Geometry check sheet. Reference: the model listing, model coordinates, mm. Face numbers are marked on the shaded views. Give positions to 0.01 mm unless a question says otherwise; leave off trailing zeros. Write each loop counter-clockwise with the first axis right and the second up, starting at its lowest first coordinate (ties: lowest second). Pieces come first, ordered by that corner, then holes. Notation, with made-up numbers: (23.25, -24.75) - (80.25, -24.75) arc R29 ccw to (80.25, 6.25) - close; hole circle Ø11 at (82.5, -18). An arc over 180 degrees is marked (long way). Use a Markdown table: item, result.
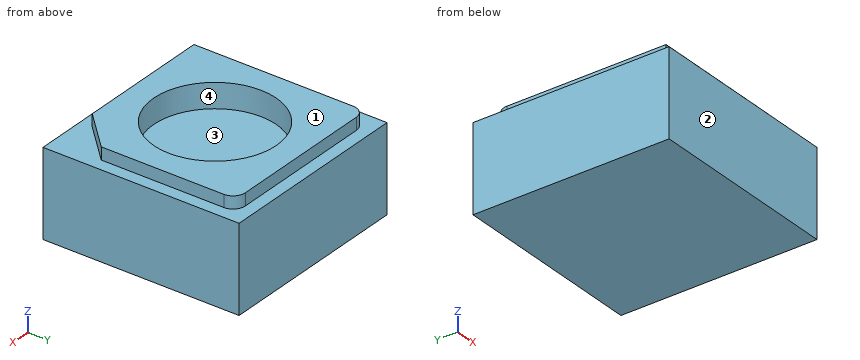
```python
from build123d import *

# Parameters (mm, degrees)
SKETCH1_W           = 80
SKETCH1_H           = 80
BOSS_EXTRUDE1_DEPTH = 35
BOSS_EXTRUDE2_START = 35
BOSS_EXTRUDE2_DEPTH = 5
CUT_EXTRUDE1_START  = 40
SKETCH3_R           = 25
CUT_EXTRUDE1_DEPTH  = 10


with BuildPart() as part:
    # Sketch1 → Boss-Extrude1 (new body)
    with BuildSketch(Plane.XY):
        with Locations((40, 40)):
            Rectangle(SKETCH1_W, SKETCH1_H)
    extrude(amount=BOSS_EXTRUDE1_DEPTH)

    # Sketch2 → Boss-Extrude2 (add)
    with BuildSketch(Plane.XY.offset(BOSS_EXTRUDE2_START)):
        with BuildLine():
            Line((60, 5), (75, 20))
            Line((75, 20), (75, 70))
            ThreePointArc((75, 70), (73.535533906, 73.535533906), (70, 75))
            Line((70, 75), (10, 75))
            ThreePointArc((10, 75), (6.464466094, 73.535533906), (5, 70))
            Line((5, 70), (5, 5))
            Line((5, 5), (60, 5))
        make_face()
    extrude(amount=BOSS_EXTRUDE2_DEPTH)

    # Sketch3 → Cut-Extrude1 (cut)
    with BuildSketch(Plane.XY.offset(CUT_EXTRUDE1_START)):
        with Locations((40, 40)):
            Circle(SKETCH3_R)
    extrude(amount=-CUT_EXTRUDE1_DEPTH, mode=Mode.SUBTRACT)


solid = part.part
```
1) Section check D-D on y = 59. Record the boundary of the cut face in (x, z).
Working result:
| item | result |
|---|---|
| outline | (0, 0) - (80, 0) - (80, 35) - (75, 35) - (75, 40) - (56.25, 40) - (56.25, 30) - (23.75, 30) - (23.75, 40) - (5, 40) - (5, 35) - (0, 35) - close |
2) Depth check by flat-ended pin: P1, Ø25, axis at x = 37, y = 41, coming from the +Z side; P2, Ø2.5, axis at x = 33, z = 38.5, coming from the +Y side; P3, Ø1.5, axis at y = 49.5, z = 36.5, coming from the -X side. Enter the tip coordinate at first touch or a pass-through.
Working result:
| item | result |
|---|---|
| P1 | stops at z = 30 |
| P2 | stops at y = 75 |
| P3 | stops at x = 5 |
3) Section check C-C on x = 11.5. Record the boundary of the cut face in (y, z).
Working result:
| item | result |
|---|---|
| outline | (0, 0) - (80, 0) - (80, 35) - (75, 35) - (75, 40) - (5, 40) - (5, 35) - (0, 35) - close |
4) Mould release check, pull along Y, two halves, no side actions. Record for the marked faces 1, 2, 3 and 4: pulls with the +Y half, pulls with the -Y half, needs draft (parallel to the pull), parting line crosses it, or undercut.
Working result:
| item | result |
|---|---|
| face 1 | needs draft |
| face 2 | pulls with the -Y half |
| face 3 | undercut |
| face 4 | undercut |
5) Section check B-B on y = 40. Record the boundary of the cut face in (x, z), then the cut area to 3 significant figures.
Working result:
| item | result |
|---|---|
| outline | (0, 0) - (80, 0) - (80, 35) - (75, 35) - (75, 40) - (65, 40) - (65, 30) - (15, 30) - (15, 40) - (5, 40) - (5, 35) - (0, 35) - close |
| area | 2,650 mm² |
6) Section check A-A on x = 67. Record the boundary of the cut face in (y, z).
Working result:
| item | result |
|---|---|
| outline | (0, 0) - (80, 0) - (80, 35) - (75, 35) - (75, 40) - (12, 40) - (12, 35) - (0, 35) - close |
7) Material ranges on L1, parallel to Y at x = 40, z = 37; L2, parallel to Z at x = 64.5, y = 39; L3, parallel to X at y = 56, z = 38.5, recorded low to high. Write a range as from..to.
Working result:
| item | result |
|---|---|
| L1 | y = 5..15, 65..75 |
| L2 | z = 0..30 |
| L3 | x = 5..20.79, 59.21..75 |
